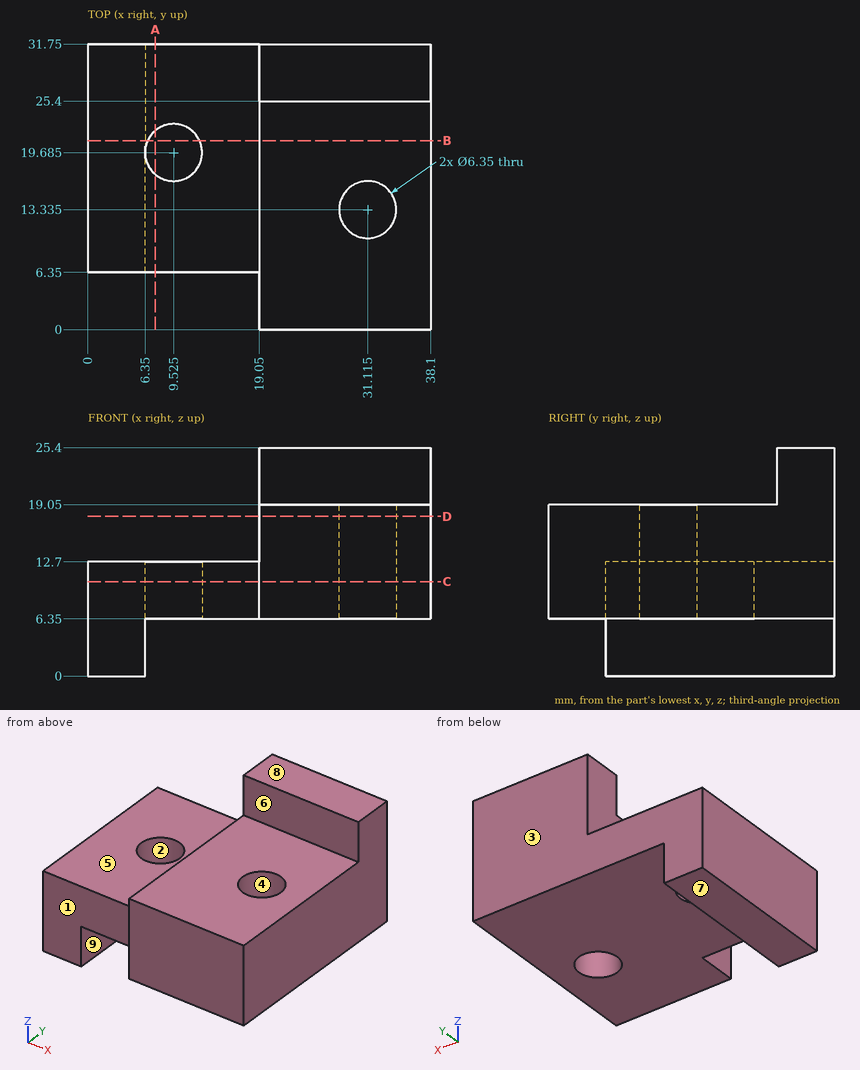
Source: three-view drawing plus pictorial views. Frame: mm from the lowest corner of the part. A direction names the side the tool comes from. Coordinates: 2 decimals unless noted, no trailing zeros. Loops run counter-clockwise (first coordinate to the right, second up) from the corner with the lowest first, then second, coordinate; pieces in that order, holes last. Notation, with made-up numbers: (42.25, 49) - (96.25, 49) arc R30 cw to (96.25, 73) - close; hole circle Ø5 at (77.5, 28.5). An arc over 180 degrees is marked (long way). Answer in a Markdown table with one row per item. Add a question column.
Item 1: Contact query for flat-ended pins moving along their axis: P1, Ø1.9, axis at y = 17.5, z = 5, coming from the +X side; P2, Ø12, axis at x = 13.5, y = 17.5, coming from the +Z side; P3, Ø5, axis at x = 22.5, y = 24.5, coming from the -Z side. Output: stop coordinate, or through.
Item 2: Section query A-A on x = 7.5. Return the cut outline in (y, z), then the cut area to 3 significant figures.
Item 3: Section query D-D on z = 17.75. Return the cut outline in (x, y) (3 decimals).
Item 4: Mould query, pull axis Y, two halves, no side actions, for the marked faces 1, 2, 3 and 4. Classes: released by +Y, released by -Y, zero draft, split by the parting line, or undercut.
Item 5: Section query B-B on y = 21. Return the cut outline in (x, z), then the cut area to 3 significant figures.
Item 6: Section query C-C on z = 10.5. Return the cut outline in (x, y) (3 decimals), then the cut area to 3 significant figures.
Item 7: Line query: line 1 along Z through (x, y) = (21, 27); line 2 along Z through (x, y) = (20, 18); line 3 along X through (y, z) = (5.5, 11.25). Output: solid intervals per line, ascending. Write a range as [from, to].
Item 8: Access query for the marked faces 5, 6, 7, 8 and 9. Directions: +Z, -Z, +X, -X, +Y, -Y. A direction counts if a zero-diameter tool reaches every point of the face in a straight line with its end or side. Return the directions, or none.
Recorded:
| question | item | result |
|---|---|---|
| 1 | P1 | x = 6.35 |
| 1 | P2 | z = 19.05 |
| 1 | P3 | z = 6.35 |
| 2 | outline | (6.35, 6.35) - (17.24, 6.35) - (17.24, 12.7) - (6.35, 12.7) - close; (22.13, 6.35) - (31.75, 6.35) - (31.75, 12.7) - (22.13, 12.7) - close |
| 2 | area | 130 mm^2 |
| 3 | outline | (19.05, 0) - (38.1, 0) - (38.1, 31.75) - (19.05, 31.75) - close; hole circle Ø6.35 at (31.115, 13.335) |
| 4 | face 1 | released by -Y |
| 4 | face 2 | undercut |
| 4 | face 3 | released by +Y |
| 4 | face 4 | undercut |
| 5 | outline | (0, 0) - (6.35, 0) - (6.35, 6.35) - (6.64, 6.35) - (6.64, 12.7) - (0, 12.7) - close; (12.41, 6.35) - (38.1, 6.35) - (38.1, 19.05) - (19.05, 19.05) - (19.05, 12.7) - (12.41, 12.7) - close |
| 5 | area | 367 mm^2 |
| 6 | outline | (0, 6.35) - (19.05, 6.35) - (19.05, 0) - (38.1, 0) - (38.1, 31.75) - (0, 31.75) - close; hole circle Ø6.35 at (9.525, 19.685); hole circle Ø6.35 at (31.115, 13.335) |
| 6 | area | 1,030 mm^2 |
| 7 | line 1 | [6.35, 25.4] |
| 7 | line 2 | [6.35, 19.05] |
| 7 | line 3 | [19.05, 38.1] |
| 8 | face 5 | +Z, -X, +Y, -Y |
| 8 | face 6 | +Z, +X, -X, -Y |
| 8 | face 7 | -Z, +X, -X, +Y, -Y |
| 8 | face 8 | +Z, +X, -X, +Y, -Y |
| 8 | face 9 | -Z, +X, +Y, -Y |
